Geometry: final body of the model. Coordinates: model frame, mm. A direction names the side the tool comes from. Round coordinates to 2 decimals unless told otherwise and drop trailing zeros. Order: outer loops, then holes, each group sorted by start corner. A loop starts at its lowest first (then second) coordinate and runs counter-clockwise, first axis right, second up. Notation, with made-up numbers: (-9.5, 14) -> (29.5, 14) arc R8 cw to (29.5, 22) -> close; hole circle Ø3 at (11.5, 51.5). An arc over 180 degrees is marked (long way). Put each result on its own line as item: value.
```python
from build123d import *

# Parameters (mm, degrees)
SKETCH_1_R               = 31.5
SKETCH_1_R_2             = 3.05
EXTRUDE_3_DEPTH          = 6
SKETCH_4_R               = 5
EXTRUDE_5_DEPTH          = 145.4
SKETCH_8_W               = 20
SKETCH_8_H               = 145.4
EXTRUDE_8_DEPTH          = 0.5
PATTERN_CIRCULAR_1_COUNT = 4
FILLET_1_R               = 10
EXTRUDE_10_DEPTH         = 3
SKETCH_11_R              = 1.6
CUT_EXTRUDE_1_DEPTH      = 3
SKETCH_12_W              = 10
SKETCH_12_H              = 45
CUT_EXTRUDE_2_DEPTH      = 3
FILLET_3_R               = 10
SKETCH_18_W              = 40
SKETCH_18_H              = 40
EXTRUDE_18_DEPTH         = 70
SKETCH_19_W              = 42
SKETCH_19_H              = 27
CUT_EXTRUDE_3_DEPTH      = 1
SKETCH_20_W              = 42
SKETCH_20_H              = 27
CUT_EXTRUDE_4_DEPTH      = 1
SKETCH_21_W              = 42
SKETCH_21_H              = 27
CUT_EXTRUDE_5_DEPTH      = 1
SKETCH_22_W              = 41
SKETCH_22_H              = 27
CUT_EXTRUDE_6_DEPTH      = 1
FILLET_4_R               = 2


with BuildPart() as part:
    # 草图1 → 凸台-拉伸3 (new body)
    with BuildSketch(Plane(origin=(0, 0, 0), x_dir=(1, 0, 0), z_dir=(0, 1, 0))):
        with Locations(Location((0, 0, 0), (0, 0, 270))):
            Circle(SKETCH_1_R)
        with Locations(Location((-17.67766953, 17.67766953, 0), (0, 0, 270))):
            Circle(SKETCH_1_R_2, mode=Mode.SUBTRACT)
        with Locations(Location((17.67766953, 17.67766953, 0), (0, 0, 270))):
            Circle(SKETCH_1_R_2, mode=Mode.SUBTRACT)
        with Locations(Location((-17.67766953, -17.67766953, 0), (0, 0, 270))):
            Circle(SKETCH_1_R_2, mode=Mode.SUBTRACT)
        with Locations(Location((17.67766953, -17.67766953, 0), (0, 0, 270))):
            Circle(SKETCH_1_R_2, mode=Mode.SUBTRACT)
    extrude(amount=EXTRUDE_3_DEPTH)

    # 草图4 → 凸台-拉伸5 (add)
    with BuildSketch(Plane.XZ):
        with Locations(Location((0, 0, 0), (0, 0, 270))):
            Circle(SKETCH_4_R)
    extrude(amount=-EXTRUDE_5_DEPTH)

    # 草图8 → 凸台-拉伸8 (add, symmetric)
    with BuildSketch(Plane(origin=(0, 0, 0), x_dir=(0, 0, -1), z_dir=(1, 0, 0))):
        with Locations((10, 72.7)):
            Rectangle(SKETCH_8_W, SKETCH_8_H)
    extrude_8 = extrude(amount=EXTRUDE_8_DEPTH, both=True)

    # 阵列(圆周)1: 凸台-拉伸8 ×4 about axis
    pattern_circular_1_axis = Axis((0, 0, 0), (0, 1, 0))
    for i in range(1, PATTERN_CIRCULAR_1_COUNT):
        add(extrude_8.rotate(pattern_circular_1_axis, i * 360 / PATTERN_CIRCULAR_1_COUNT))

    # 圆角1
    fillet_1_edges = [part.edges().sort_by_distance(p)[0] for p in [
        (-3.535533906, 6, -3.535533906),
        (-3.535533906, 6, 3.535533906),
        (3.535533906, 6, 3.535533906),
        (3.535533906, 6, -3.535533906),
    ]]
    fillet(fillet_1_edges, radius=FILLET_1_R)

    # 草图10 → 凸台-拉伸10 (add)
    with BuildSketch(Plane(origin=(0, 145.4, 0), x_dir=(1, 0, 0), z_dir=(0, 1, 0))):
        with BuildLine():
            Line((-37.499452899, -27.999452899), (37.499452899, -27.999452899))
            ThreePointArc((37.499452899, -27.999452899), (39.620773242, -27.120773242), (40.499452899, -24.999452899))
            Line((40.499452899, -24.999452899), (40.499452899, 24.999452899))
            ThreePointArc((40.499452899, 24.999452899), (39.620773242, 27.120773242), (37.499452899, 27.999452899))
            Line((37.499452899, 27.999452899), (-37.499452899, 27.999452899))
            ThreePointArc((-37.499452899, 27.999452899), (-39.620773242, 27.120773242), (-40.499452899, 24.999452899))
            Line((-40.499452899, 24.999452899), (-40.499452899, -24.999452899))
            ThreePointArc((-40.499452899, -24.999452899), (-39.620773242, -27.120773242), (-37.499452899, -27.999452899))
        make_face()
    extrude(amount=EXTRUDE_10_DEPTH)

    # 草图11 → 切除-拉伸1 (cut)
    with BuildSketch(Plane(origin=(0, 148.4, 0), x_dir=(1, 0, 0), z_dir=(0, 1, 0))):
        with Locations(Location((-37.499452899, 24.999452899, 0), (0, 0, 270))):
            Circle(SKETCH_11_R)
        with Locations(Location((-37.499452899, -24.999452899, 0), (0, 0, 270))):
            Circle(SKETCH_11_R)
        with Locations(Location((37.499452899, 24.999452899, 0), (0, 0, 270))):
            Circle(SKETCH_11_R)
        with Locations(Location((37.499452899, -24.999452899, 0), (0, 0, 270))):
            Circle(SKETCH_11_R)
    extrude(amount=-CUT_EXTRUDE_1_DEPTH, mode=Mode.SUBTRACT)

    # 草图12 → 切除-拉伸2 (cut)
    with BuildSketch(Plane(origin=(0, 148.4, 0), x_dir=(1, 0, 0), z_dir=(0, 1, 0))):
        with Locations((-35.499452899, 0)):
            Rectangle(SKETCH_12_W, SKETCH_12_H)
    extrude(amount=-CUT_EXTRUDE_2_DEPTH, mode=Mode.SUBTRACT)

    # 圆角3
    fillet_3_edges = [part.edges().sort_by_distance(p)[0] for p in [
        (3.535533906, 145.4, -3.535533906),
        (3.535533906, 145.4, 3.535533906),
        (-3.535533906, 145.4, 3.535533906),
        (-3.535533906, 145.4, -3.535533906),
    ]]
    fillet(fillet_3_edges, radius=FILLET_3_R)

    # 草图18 → 凸台-拉伸18 (add)
    with BuildSketch(Plane(origin=(0, 148.4, 0), x_dir=(1, 0, 0), z_dir=(0, 1, 0))):
        Polygon((-20, 21), (-21, 20), (-21, -20), (-20, -21), (20, -21), (21, -20), (21, 20), (20, 21), align=None)
        Rectangle(SKETCH_18_W, SKETCH_18_H, mode=Mode.SUBTRACT)
    extrude(amount=-EXTRUDE_18_DEPTH)

    # 草图19 → 切除-拉伸3 (cut)
    with BuildSketch(Plane(origin=(21, 0, 0), x_dir=(0, 0, -1), z_dir=(1, 0, 0))):
        with Locations((0, 131.9)):
            Rectangle(SKETCH_19_W, SKETCH_19_H)
    extrude(amount=-CUT_EXTRUDE_3_DEPTH, mode=Mode.SUBTRACT)

    # 草图20 → 切除-拉伸4 (cut)
    with BuildSketch(Plane(origin=(0, 0, -21), x_dir=(-1, 0, 0), z_dir=(0, 0, -1))):
        with Locations((0, 131.9)):
            Rectangle(SKETCH_20_W, SKETCH_20_H)
    extrude(amount=-CUT_EXTRUDE_4_DEPTH, mode=Mode.SUBTRACT)

    # 草图21 → 切除-拉伸5 (cut)
    with BuildSketch(Plane.ZY.offset(21)):
        with Locations((0, 131.9)):
            Rectangle(SKETCH_21_W, SKETCH_21_H)
    extrude(amount=-CUT_EXTRUDE_5_DEPTH, mode=Mode.SUBTRACT)

    # 草图22 → 切除-拉伸6 (cut)
    with BuildSketch(Plane.XY.offset(21)):
        with Locations((-0.5, 131.9)):
            Rectangle(SKETCH_22_W, SKETCH_22_H)
    extrude(amount=-CUT_EXTRUDE_6_DEPTH, mode=Mode.SUBTRACT)

    # 圆角4
    fillet_4_edges = [part.edges().sort_by_distance(p)[0] for p in [
        (20, 98.4, -0.5),
        (20, 98.4, 0.5),
        (0.5, 98.4, -20),
        (-0.5, 98.4, -20),
        (-20, 98.4, -0.5),
        (-20, 98.4, 0.5),
        (-0.5, 98.4, 20),
        (0.5, 98.4, 20),
    ]]
    fillet(fillet_4_edges, radius=FILLET_4_R)


solid = part.part
```
1. Material intervals for probe 1 along X at (y, z) = (102.5, 15.5); probe 2 along Y at (x, z) = (-18, 23), sorted ascending.
Ans:
probe 1: -21 to -20, -0.5 to 0.5, 20 to 21
probe 2: 0 to 6, 145.4 to 148.4
2. Set-up query: faces 3 (the face through (-20.1, 118.4, 1.7)), 4 (the face through (1, 147, -27.999)), 5 (the face through (-36, 147, 22.5)), 6 (the face through (-15.106, 2.958, -16.038)). Return all of +Z, -Z, +X, -X, +Y, -Y with unobstructed straight access to the full face (end or side cutting, diameter ignored); none if empty.
Ans:
face 3: none
face 4: -Z, +X, -X, +Y
face 5: -X, +Y, -Y
face 6: -Y
3. Contact query for flat-ended pins moving along their axis: P1, Ø0.8, axis at y = 43.5, z = 0, coming from the +X side; P2, Ø8, axis at y = 112, z = 4.5, coming from the -X side; P3, Ø7.5, axis at x = 14.5, y = 101.5, coming from the +Z side; P4, Ø3, axis at x = -37.5, z = -25, coming from the +Y side. Output: stop coordinate, or through.
Ans:
P1: x = 20
P2: x = -21
P3: z = 21
P4: through
4. Cut plane B-B on y = 90. State how many separate pieces and enclosed holes the cut face has, and give its area (3 significant figures).
Ans:
separate pieces: 1
enclosed holes: 4
area: 307 mm²
5. Draft query along Y for faces 1 (the face through (-3.57, 74.86, -3.5)), 2 (the face through (-39.6, 146.88, -27.14)). Return one class per face: +Y half, -Y half, draft (parallel to the pull), parting line (faces both ways), or undercut.
Ans:
face 1: undercut
face 2: draft
6. Cut plane A-A on y = 56. Return loops of the section in (x, z).
Ans:
outline: (-20, -0.5) -> (-4.97, -0.5) arc R5 ccw to (-0.5, -4.97) -> (-0.5, -20) -> (0.5, -20) -> (0.5, -4.97) arc R5 ccw to (4.97, -0.5) -> (20, -0.5) -> (20, 0.5) -> (4.97, 0.5) arc R5 ccw to (0.5, 4.97) -> (0.5, 20) -> (-0.5, 20) -> (-0.5, 4.97) arc R5 ccw to (-4.97, 0.5) -> (-20, 0.5) -> close
